Autodesk Inventor part; units mm, degrees
ref_plane "YZ Plane" through (0, 0, 0) normal (1, 0, 0) x (0, 1, 0)
ref_plane "XZ Plane" through (0, 0, 0) normal (0, 1, 0) x (-1, 0, 0)
ref_plane "XY Plane" through (0, 0, 0) normal (0, 0, 1) x (1, 0, 0)
sketch "Sketch_9" plane through (0, 0, 0) normal (0, 0, 1) x (1, 0, 0)
  line L0 (50, 0) -> (-50, 0)
  line L1 (0, 23.2) -> (0, 22.2)
  line L2 (0, 22.2) -> (0.15, 22.2)
  arc A0 (0.45, 21.9) -> (0.15, 22.2) centre (0.15, 21.9) ccw
  line L3 (0.45, 21.9) -> (0.45, 21.6)
  line L4 (0.45, 21.6) -> (2.3864, 21.6)
  arc A1 (4.6136, 21.6) -> (2.3864, 21.6) centre (3.5, 20.25) ccw
  line L5 (4.6136, 21.6) -> (6.55, 21.6)
  line L6 (6.55, 21.6) -> (6.55, 21.9)
  arc A2 (6.85, 22.2) -> (6.55, 21.9) centre (6.85, 21.9) ccw
  line L7 (6.85, 22.2) -> (7, 22.2)
  line L8 (7, 22.2) -> (7, 23.2)
  arc A3 (7, 23.2) -> (6.7, 23.5) centre (6.7, 23.2) ccw
  line L9 (6.7, 23.5) -> (0.3, 23.5)
  arc A4 (0.3, 23.5) -> (0, 23.2) centre (0.3, 23.2) ccw
revolve "Revolution1" add sketch "Sketch_9" angle 360 about axis through (50, 0, 0) along (1, 0, 0)
properties part number "61807-2RS1_PART2" material "Stainless Steel"
Can you work these out from the model? Positions are in its coordinate system, mm. Coordinates: 2 decimals unless noted, no trailing zeros. Loops run counter-clockwise (first coordinate to the right, second up) from the corner with the lowest first, then second, coordinate; pieces in that order, holes last. Notation, with made-up numbers: (11.5, 67.25) -> (30.5, 67.25) arc R24 cw to (30.5, 81.25) -> close; hole circle Ø5 at (-24, 37.25). An arc over 180 degrees is marked (long way). Answer as a JSON object with one key per item and string values.
1) If I drill on line 1 (Z direction, x = 1, y = 0); line 2 (Y direction, x = 5, z = 18), over which ranges is the centre line in solid material (lowest first)?
Results:
{"line 1": "z = -23.5 to -21.6, 21.6 to 23.5", "line 2": "y = -15.11 to -11.94, 11.94 to 15.11"}
2) Thinking about a two-plate mould opening in Z: for faces 1 (the face through (5.595, -4.682, -21.086)), 2 (the face through (0, 19, -12)), 3 (the face through (3.5, 22.4, -7.1)), 4 (the face through (1.432, -4.682, -21.086)), which applies, pulls with the +Z half, pulls with the -Z half, needs draft (parallel to the pull), parting line crosses it, or undercut?
Results:
{"face 1": "undercut", "face 2": "needs draft", "face 3": "parting line crosses it", "face 4": "undercut"}
3) For P1, Ø4, axis at x = 4, y = -12.5, coming from the +Z side; P2, Ø12, axis at y = -6.5, z = -9, coming from the -X side, each with a flat end and sliding along its axis, tell me the tip position at first contact or that it passes through.
Results:
{"P1": "stops at z = 21.02", "P2": "passes through"}
4) Imagine slicing it at A-A (y = 0). Please give me the cut outline in (x, z).
Results:
{"outline": "(0, -23.2) arc R0.3 ccw to (0.3, -23.5) -> (6.7, -23.5) arc R0.3 ccw to (7, -23.2) -> (7, -22.2) -> (6.85, -22.2) arc R0.3 cw to (6.55, -21.9) -> (6.55, -21.6) -> (4.61, -21.6) arc R1.75 cw to (2.39, -21.6) -> (0.45, -21.6) -> (0.45, -21.9) arc R0.3 cw to (0.15, -22.2) -> (0, -22.2) -> close; (0, 22.2) -> (0.15, 22.2) arc R0.3 cw to (0.45, 21.9) -> (0.45, 21.6) -> (2.39, 21.6) arc R1.75 cw to (4.61, 21.6) -> (6.55, 21.6) -> (6.55, 21.9) arc R0.3 cw to (6.85, 22.2) -> (7, 22.2) -> (7, 23.2) arc R0.3 ccw to (6.7, 23.5) -> (0.3, 23.5) arc R0.3 ccw to (0, 23.2) -> close"}
5) Imagine slicing it at C-C (x = 3). Please give me the cut outline in (y, z).
Results:
{"outline": "circle Ø47 at (0, 0); hole circle Ø43.85 at (0, 0)"}
